```python
from build123d import *

# Parameters (mm, degrees)
EXTRUDE_1_DEPTH     = 8
SKETCH_2_R          = 2
CUT_EXTRUDE_2_DEPTH = 22.400934559
SKETCH_3_R          = 2
CUT_EXTRUDE_1_DEPTH = 27.033270693
CHAMFER_1_SIZE      = 2


with BuildPart() as part:
    # Эскиз1 → Вытянуть1 (new body)
    with BuildSketch(Plane.XY):
        Polygon((-13, 15), (13, 15), (13, 6.500000002), (6.716266963, 6.500000002), (6.716266963, -8.894499905), (2, -8.894499905), (2, 0.42128884), (-2, 0.42128884), (-2, -8.894499905), (-6.716266963, -8.894499905), (-6.716266963, 6.500000002), (-13, 6.500000002), align=None)
    extrude(amount=EXTRUDE_1_DEPTH)

    # Эскиз2 → Вытянуть2 (cut, through all)
    with BuildSketch(Plane.XY.offset(8)):
        with Locations((-8, 10.748498226)):
            Circle(SKETCH_2_R)
        with Locations((8, 10.750000001)):
            Circle(SKETCH_2_R)
    extrude(amount=-CUT_EXTRUDE_2_DEPTH, mode=Mode.SUBTRACT)

    # Эскиз3 → Вырез-Вытянуть1 (cut, through all)
    with BuildSketch(Plane(origin=(6.716266963, 0, 0), x_dir=(0, 0, -1), z_dir=(1, 0, 0))):
        with Locations((-4, -4.14834478)):
            Circle(SKETCH_3_R)
    extrude(amount=-CUT_EXTRUDE_1_DEPTH, mode=Mode.SUBTRACT)

    # Фаска1
    chamfer_1_edges = [part.edges().sort_by_distance(p)[0] for p in [
        (4.358133481, -8.894499905, 0),
        (-4.358133481, -8.894499905, 0),
        (-4.358133481, -8.894499905, 8),
        (4.358133481, -8.894499905, 8),
    ]]
    chamfer(chamfer_1_edges, length=CHAMFER_1_SIZE)


solid = part.part
```
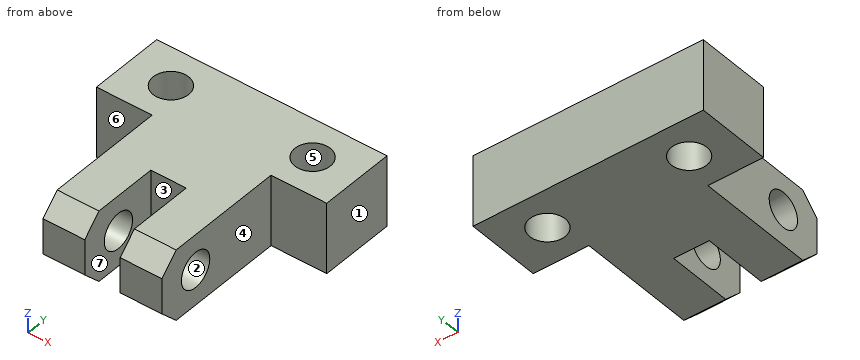
Work out the finished part from the listing and answer in its coordinate system (mm). Face numbers are marked on the shaded views. A direction names the side the tool comes from. Round coordinates to 2 decimals unless told otherwise and drop trailing zeros. Write each loop counter-clockwise with the first axis right and the second up, starting at its lowest first coordinate (ties: lowest second). Pieces come first, ordered by that corner, then holes.
1) A cutting plane is placed at B-B on z = 4.25. Determine the outline of the cut face in (x, y), and give its area (3 significant figures).
2) Consider probe 1 along X at (y, z) = (-0.25, 3.75); probe 2 along Y at (x, z) = (3.7, 4); probe 3 along X at (y, z) = (12.5, 5.5). Determine where each line is inside the solid, lowest interval first.
3) A cutting plane is placed at D-D on z = 1.5. Determine the outline of the cut face in (x, y).
4) Which of the six approach directions +Z, -Z, +X, -X, +Y, -Y give full straight-line access (tool end or side, diameter ignored) to the marked faces 4, 5, 6 and 7?
5) Determine the mould class of the marked faces 1, 2 and 3 for opening direction X: pulls with the +X half, pulls with the -X half, needs draft (parallel to the pull), parting line crosses it, or undercut.
6) A cutting plane is placed at C-C on y = 11.75. Determine the outline of the cut face in (x, z), and give its area (3 significant figures).
7) A flat-ended cylindrical pin translates along its axis: P1, Ø3, axis at x = -8.5, z = 5.5, coming from the -Y side. Find the tip coordinate at first contact, or state that the pin passes through.
8) A cutting plane is placed at A-A on x = 8. Determine the outline of the cut face in (y, z), and give its area (3 significant figures).
Entries:
1. outline: (-13, 6.5) - (-6.72, 6.5) - (-6.72, -2.16) - (-2, -2.16) - (-2, 0.42) - (2, 0.42) - (2, -2.16) - (6.72, -2.16) - (6.72, 6.5) - (13, 6.5) - (13, 15) - (-13, 15) - close; (-6.72, -8.89) - (-2, -8.89) - (-2, -6.13) - (-6.72, -6.13) - close; (2, -8.89) - (6.72, -8.89) - (6.72, -6.13) - (2, -6.13) - close; hole circle Ø4 at (-8, 10.75); hole circle Ø4 at (8, 10.75)
1. area: 328 mm2
2. probe 1: x = -6.72 to -2, 2 to 6.72
2. probe 2: y = -8.89 to -6.15, -2.15 to 15
2. probe 3: x = -13 to -8.97, -7.03 to 7.03, 8.97 to 13
3. outline: (-13, 6.5) - (-6.72, 6.5) - (-6.72, -8.39) - (-2, -8.39) - (-2, 0.42) - (2, 0.42) - (2, -8.39) - (6.72, -8.39) - (6.72, 6.5) - (13, 6.5) - (13, 15) - (-13, 15) - close; hole circle Ø4 at (-8, 10.75); hole circle Ø4 at (8, 10.75)
4. face 4: +Z, -Z, +X, -Y
4. face 5: +Z, -Z
4. face 6: +Z, -Z, -X, -Y
4. face 7: +Z, -Z, -Y
5. face 1: pulls with the +X half
5. face 2: needs draft
5. face 3: undercut
6. outline: (-13, 0) - (-9.73, 0) - (-9.73, 8) - (-13, 8) - close; (-6.27, 0) - (6.27, 0) - (6.27, 8) - (-6.27, 8) - close; (9.73, 0) - (13, 0) - (13, 8) - (9.73, 8) - close
6. area: 153 mm2
7. P1: stops at y = 6.5
8. outline: (6.5, 0) - (8.75, 0) - (8.75, 8) - (6.5, 8) - close; (12.75, 0) - (15, 0) - (15, 8) - (12.75, 8) - close
8. area: 36.0 mm2
